Geometry check sheet. Reference: the model listing, model coordinates, mm. Face numbers are marked on the shaded views. A direction names the side the tool comes from. Coordinates: 2 decimals unless noted, no trailing zeros. Loops run counter-clockwise (first coordinate to the right, second up) from the corner with the lowest first, then second, coordinate; pieces in that order, holes last. Notation, with made-up numbers: (83.5, 80) -> (99.5, 80) arc R22 cw to (99.5, 93) -> close; hole circle Ø11 at (48.5, -32). An arc over 180 degrees is marked (long way). Answer as a JSON object with one key per item and string values.
from build123d import *

# Parameters (mm, degrees)
SKETCH1_W           = 11.43
SKETCH1_H           = 9.525
BOSS_EXTRUDE1_DEPTH = 88.9
SKETCH2_R           = 3.175
BOSS_EXTRUDE2_DEPTH = 130.175


with BuildPart() as part:
    # Sketch1 → Boss-Extrude1 (new body)
    with BuildSketch(Plane(origin=(0, 0, 0), x_dir=(0, 0, -1), z_dir=(1, 0, 0))):
        Rectangle(SKETCH1_W, SKETCH1_H)
    extrude(amount=BOSS_EXTRUDE1_DEPTH)

    # Sketch2 → Boss-Extrude2 (add)
    with BuildSketch(Plane.XZ.offset(4.7625)):
        with Locations((44.45, 0)):
            Circle(SKETCH2_R)
    extrude(amount=BOSS_EXTRUDE2_DEPTH)


solid = part.part
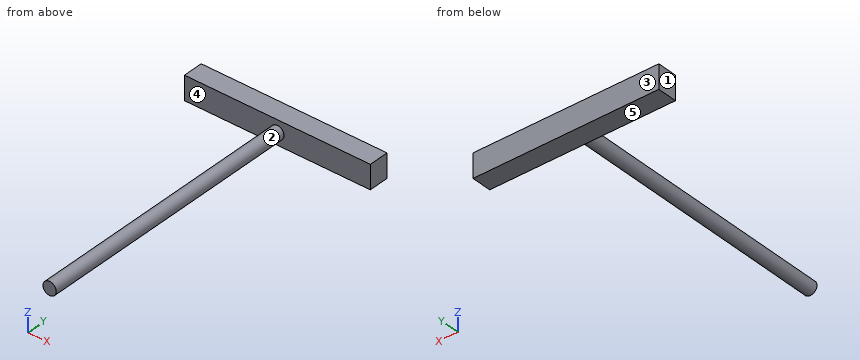
1. Section check D-D, the plane x = 7. Record the boundary of the cut face in (y, z) (1 decimal), then the cut area to 3 significant figures.
Evaluation:
{"outline": "(-4.8, -5.7) -> (4.8, -5.7) -> (4.8, 5.7) -> (-4.8, 5.7) -> close", "area": "109 mm^2"}
2. Section check A-A, the plane z = 0. Record the boundary of the cut face in (x, y) (1 decimal), then the cut area to 3 significant figures.
Evaluation:
{"outline": "(0, -4.8) -> (41.3, -4.8) -> (41.3, -134.9) -> (47.6, -134.9) -> (47.6, -4.8) -> (88.9, -4.8) -> (88.9, 4.8) -> (0, 4.8) -> close", "area": "1,670 mm^2"}
3. Tool access check on the marked faces 1 and 2. Record the directions out of +Z, -Z, +X, -X, +Y, -Y that give a thin tool (end or side, any length) a straight path to the whole face; none if there is none.
Evaluation:
{"face 1": "+Z, -Z, -X, +Y, -Y", "face 2": "-Y"}
4. Section check C-C, the plane y = -109. Record the boundary of the cut face in (x, z) (3 decimals).
Evaluation:
{"outline": "circle Ø6.35 at (44.45, 0)"}
5. Mould release check, pull along Y, two halves, no side actions. Record for the marked faces 3, 4 and 5: released by +Y, released by -Y, zero draft, split by the parting line, or undercut.
Evaluation:
{"face 3": "released by +Y", "face 4": "released by -Y", "face 5": "zero draft"}
6. Thickness scan on probe 1 along Y at (x, z) = (48.5, 3.5); probe 2 along X at (y, z) = (-18, -1.75); probe 3 along X at (y, z) = (-50.5, 2.25). Record the ranges inside material, lowest first. Write a range as from..to.
Evaluation:
{"probe 1": "y = -4.76..4.76", "probe 2": "x = 41.8..47.1", "probe 3": "x = 42.21..46.69"}
7. Section check B-B, the plane x = 44.45. Record the boundary of the cut face in (y, z) (1 decimal), then the cut area to 3 significant figures.
Evaluation:
{"outline": "(-134.9, -3.2) -> (-4.8, -3.2) -> (-4.8, -5.7) -> (4.8, -5.7) -> (4.8, 5.7) -> (-4.8, 5.7) -> (-4.8, 3.2) -> (-134.9, 3.2) -> close", "area": "935 mm^2"}
8. Depth check by flat-ended pin: P1, Ø3, axis at x = 52, z = 1.5, coming from the -Y side; P2, Ø6, axis at x = 43.5, y = -73, coming from the -Z side (3 decimals). Enter the tip coordinate at first touch or a pass-through.
Evaluation:
{"P1": "stops at y = -4.76", "P2": "stops at z = -3.175"}
